from build123d import *

# Parameters (mm, degrees)
SKETCH2_R           = 7
SKETCH2_R_2         = 4
BOSS_EXTRUDE2_DEPTH = 2
BOSS_EXTRUDE4_START = -2
BOSS_EXTRUDE4_DEPTH = 4


with BuildPart() as part:
    # Sketch2 → Boss-Extrude2 (new body)
    # profile 1 of 3: a face of its own
    with BuildSketch(Plane(origin=(0, 0, 0), x_dir=(1, 0, 0), z_dir=(0, 1, 0))):
        with BuildLine():
            Line((-152, 6), (-152, -6))
            Line((-152, -6), (-20, -6))
            ThreePointArc((-20, -6), (-19.650225915, -5.99529369), (-19.300451831, -6))
            Line((-19.300451831, -6), (19.300451831, -6))
            ThreePointArc((19.300451831, -6), (19.650225915, -5.99529369), (20, -6))
            Line((20, -6), (152, -6))
            Line((152, -6), (152, 6))
            Line((152, 6), (-152, 6))
        make_face()
    # profile 2 of 3: a face of its own
    with BuildSketch(Plane(origin=(0, 0, 0), x_dir=(1, 0, 0), z_dir=(0, 1, 0))):
        with BuildLine():
            Line((19.300451831, -6), (-19.300451831, -6))
            ThreePointArc((-19.300451831, -6), (-11.449616182, -8.908173189), (-7, -16))
            ThreePointArc((-7, -16), (0, -9), (7, -16))
            ThreePointArc((7, -16), (11.449616182, -8.908173189), (19.300451831, -6))
        make_face()
    # profile 3 of 3: a face of its own
    with BuildSketch(Plane(origin=(0, 0, 0), x_dir=(1, 0, 0), z_dir=(0, 1, 0))):
        with Locations((0, -16)):
            Circle(SKETCH2_R)
        with Locations(Location((0, -16, 0), (0, 0, 270))):
            Circle(SKETCH2_R_2, mode=Mode.SUBTRACT)
    extrude(amount=-BOSS_EXTRUDE2_DEPTH)

    # Boss-Extrude4: read off the stored shape, not the designer's step
    # Boss-Extrude4 outline → Boss-Extrude4 (add)
    with BuildSketch(Plane(origin=(0, 0, 0), x_dir=(1, 0, 0), z_dir=(0, 1, 0)).offset(BOSS_EXTRUDE4_START)):
        with BuildLine():
            Line((-152, 6), (-152, -6))
            Line((-152, -6), (152, -6))
            Line((152, -6), (152, 6))
            Line((152, 6), (150, 6))
            Line((150, 6), (150, -2))
            ThreePointArc((150, -2), (149.414213562, -3.414213562), (148, -4))
            Line((148, -4), (-148, -4))
            ThreePointArc((-148, -4), (-149.414213562, -3.414213562), (-150, -2))
            Line((-150, -2), (-150, 6))
            Line((-150, 6), (-152, 6))
        make_face()
    extrude(amount=BOSS_EXTRUDE4_DEPTH)


solid = part.part
Here's how the part is built. I have some questions about the finished solid (model axes, mm). A direction names the side the tool comes from. Coordinates: 2 decimals unless noted, no trailing zeros. Write each loop counter-clockwise with the first axis right and the second up, starting at its lowest first coordinate (ties: lowest second). Pieces come first, ordered by that corner, then holes.
1) If we section it at C-C (x = 86.5): List the corners of the cut face in (y, z) for me, plus the area to 3 significant figures.
Filled in:
outline: (-2, -6) - (0, -6) - (0, 4) - (2, 4) - (2, 6) - (-2, 6) - close
area: 28.0 mm2
2) Thinking about a two-plate mould opening in X: for faces 4 (the face through (11.36, -0.99, 8.98)), 5 (the face through (0, -1, 12)), 6 (the face through (0, -1, 23)), which applies, +X half, -X half, draft (parallel to the pull), parting line (faces both ways), or undercut?
Filled in:
face 4: +X half
face 5: undercut
face 6: parting line
3) If we section it at A-A (y = -1.4): List the corners of the cut face in (x, z) for me.
Filled in:
outline: (-152, -6) - (152, -6) - (152, 6) - (19.3, 6) arc R13 cw to (7, 16) arc R7 ccw to (-7, 16) arc R13 cw to (-19.3, 6) - (-152, 6) - close; hole circle Ø8 at (0, 16)
4) Which directions (+Z, -Z, +X, -X, +Y, -Y) give clear straight access to the entire face, cutting with the end or side of a thin tool? Please do faces 1 (the face through (-2, -2, 2)), 2 (the face through (-2, 0, -1)), 3 (the face through (0, 0, 11)).
Filled in:
face 1: +Z, -Z, +X, -X, -Y
face 2: -Z, +Y
face 3: +Z, +X, -X, +Y
5) I'm going to push flat-ended pins straight in: pin 1 (10.5 mm diameter, centred on x = 0, z = 16, fed in from -Y); pin 2 (1.5 mm diameter, centred on y = -0.5, z = 17, fed in from +X); pin 3 (3 mm diameter, centred on x = -74.5, z = 1, fed in from +Y). Where does each tip first touch, or does it pass through?
Filled in:
pin 1: stops at y = -2
pin 2: stops at x = 7
pin 3: stops at y = 0
6) If we section it at B-B (x = 0): List the corners of the cut face in (y, z) for me.
Filled in:
outline: (-2, -6) - (0, -6) - (0, 4) - (2, 4) - (2, 6) - (0, 6) - (0, 12) - (-2, 12) - close; (-2, 20) - (0, 20) - (0, 23) - (-2, 23) - close
7) If I drill on line 1 (X direction, y = -1.05, z = 16); line 2 (X direction, y = 0.85, z = 1.75); line 3 (Y direction, x = 49, z = -1), over which ranges is the centre line in solid material (lowest first)?
Filled in:
line 1: x = -7 to -4, 4 to 7
line 2: x = -152 to -150, 150 to 152
line 3: y = -2 to 0
